Geometry check sheet. Reference: the model listing, model coordinates, mm. Face numbers are marked on the shaded views. Round coordinates to 2 decimals unless told otherwise and drop trailing zeros. Order: outer loops, then holes, each group sorted by start corner. A loop starts at its lowest first (then second) coordinate and runs counter-clockwise, first axis right, second up.
(1) Material ranges on line 1 along X through (y, z) = (179, -3.5); line 2 along X through (y, z) = (71, 77.5); line 3 along Z through (x, y) = (0, 138), recorded low to high.
(2) Sectioned sample at B-B (z = -14.5). Record the boundary of the cut face in (x, y), plus the area to 3 significant figures.
(3) Release check for a two-part mould opening along X. For the marked faces 1 and 2 record: +X half, -X half, draft (parallel to the pull), parting line (faces both ways), or undercut.
(4) Sectioned sample at D-D (y = 180). Record the boundary of the cut face in (x, z), plus the area to 3 significant figures.
(5) Sectioned sample at A-A (x = 0). Record the boundary of the cut face in (y, z), plus the area to 3 significant figures.
(6) Go/stop test with flat-tipped pins: pin 1 (2 mm diameter, centred on y = 115, z = 49, fed in from +X); pin 2 (12 mm diameter, centred on x = 65.5, y = 116, fed in from -Z); pin 3 (2 mm diameter, centred on x = 8.5, y = 36, fed in from +Z); pin 4 (1.7 mm diameter, centred on x = 0.5, z = 101, fed in from -Y). Record where each tip stops, or that it passes through.
(7) Sectioned sample at C-C (x = -70.5). Record the boundary of the cut face in (y, z).
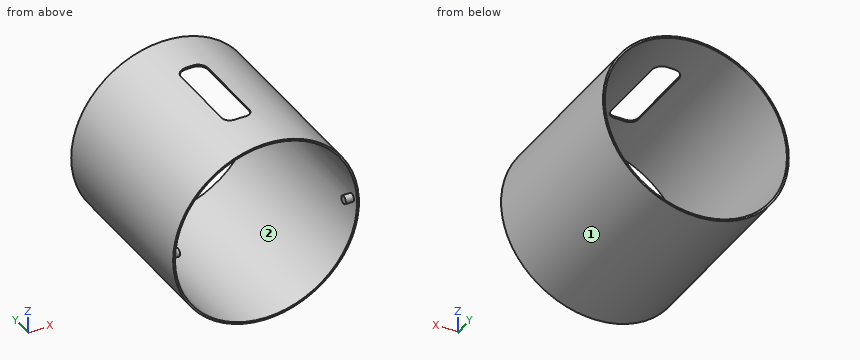
Autodesk Inventor part; units mm, degrees
ref_plane "Work Plane1" through (-101, 0, 0) normal (1, 0, 0) x (0, 1, 0)
ref_plane "XZ Plane" through (0, 0, 0) normal (0, 1, 0) x (-1, 0, 0)
ref_plane "XY Plane" through (0, 0, 0) normal (0, 0, 1) x (1, 0, 0)
sketch "Sketch1" plane through (0, 0, 0) normal (0, 1, 0) x (-1, 0, 0)
  circle A0 centre (0, 0) radius 100
  circle A1 centre (0, 0) radius 102
  dimension "d0" = 200
  dimension "d1" = 2
extrude "Extrusion1" add sketch "Sketch1" along normal blind 200
sketch "Sketch2" plane through (0, 0, 0) normal (0, 0, 1) x (1, 0, 0)
  line L0 (-5, 50) -> (0, 50)
  line L1 (0, 150) -> (-5, 150)
  line L2 (-15, 140) -> (-15, 60)
  line L3 (102, 200) -> (-102, 200)
  line L4 (0, 200) -> (0, 0) construction
  line L5 (102, 0) -> (-102, 0)
  line L6 (-102, 200) -> (102, 0) construction
  line L7 (102, 200) -> (0, 100) construction
  line L8 (0, 100) -> (-15, 100) construction
  line L9 (5, 50) -> (0, 50)
  line L10 (0, 150) -> (5, 150)
  line L11 (15, 140) -> (15, 60)
  arc A0 (-5, 150) -> (-15, 140) centre (-5, 140) ccw
  arc A1 (15, 140) -> (5, 150) centre (5, 140) ccw
  arc A2 (-15, 60) -> (-5, 50) centre (-5, 60) ccw
  arc A3 (5, 50) -> (15, 60) centre (5, 60) ccw
  point P0 (-15, 50)
  point P1 (-15, 150)
  point P2 (15, 50)
  point P3 (15, 150)
  dimension "d4" = 15
  dimension "d5" = 100
  dimension "d9" = 10
extrude "Extrusion2" cut sketch "Sketch2" along normal through all
ref_plane "Work Plane1" through (-101, 0, 0) normal (1, 0, 0) x (0, 1, 0)
sketch "Sketch3" plane through (-101, 0, 0) normal (1, 0, 0) x (0, 1, 0)
  circle A0 centre (10.5, 0) radius 4.5
  line L0 (0, 0) -> (200, 0) construction
  line L1 (200, -102) -> (200, 102)
  dimension "d11" = 9
  dimension "d12" = 10.5
extrude "Extrusion3" add sketch "Sketch3" along normal blind 10
pattern_circular "Circular Pattern1" count 2 over 360 about axis through (0, 0, 0) along (0, 1, 0) of "Extrusion3"
properties part number "cover"
Answer below:
1. line 1: x = -101.94 to -99.94, 99.94 to 101.94
1. line 2: x = -66.32 to -63.2, 63.2 to 66.32
1. line 3: z = -102 to -100
2. outline: (-100.96, 0) - (-98.94, 0) - (-98.94, 200) - (-100.96, 200) - close; (98.94, 0) - (100.96, 0) - (100.96, 200) - (98.94, 200) - close
2. area: 808 mm2
3. face 1: parting line
3. face 2: undercut
4. outline: circle Ø204 at (0, 0); hole circle Ø200 at (0, 0)
4. area: 1,270 mm2
5. outline: (0, -102) - (200, -102) - (200, -100) - (0, -100) - close; (0, 100) - (50, 100) - (50, 102) - (0, 102) - close; (150, 100) - (200, 100) - (200, 102) - (150, 102) - close
5. area: 600 mm2
6. pin 1: stops at x = 90
6. pin 2: stops at z = -82.85
6. pin 3: stops at z = 101.72
6. pin 4: stops at y = 0
7. outline: (0, -73.71) - (200, -73.71) - (200, -70.92) - (0, -70.92) - close; (0, 70.92) - (200, 70.92) - (200, 73.71) - (0, 73.71) - close
